CAD build for the part. Positions are in the model's coordinates, mm. Give positions to 0.01 mm unless a question says otherwise; leave off trailing zeros. Write each loop counter-clockwise with the first axis right and the second up, starting at its lowest first coordinate (ties: lowest second). Pieces come first, ordered by that corner, then holes. Notation, with made-up numbers: (-6.5, -22.75) - (40.5, -22.75) arc R25 cw to (40.5, 12.25) - close; hole circle Ø5 at (5, 49). An arc over 180 degrees is marked (long way). Answer as a JSON object with one key per item and string values.
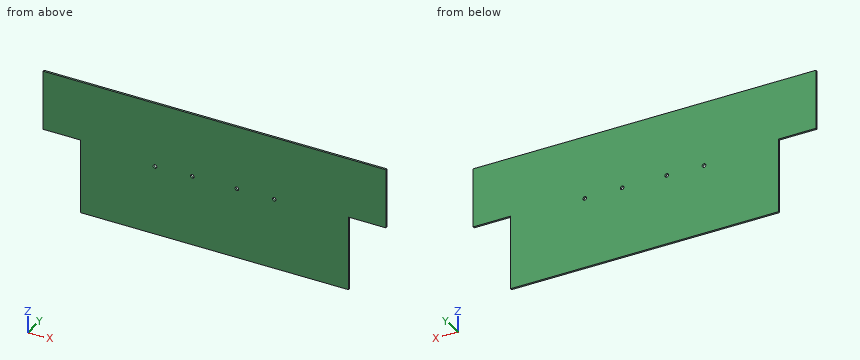
from build123d import *

# Parameters (mm, degrees)
BOSS_EXTRUDE1_DEPTH         = 3.175
F_1_4_0_25_DIAMETER_HOLE1_D = 6.35


with BuildPart() as part:
    # Sketch1 → Boss-Extrude1 (new body)
    with BuildSketch(Plane.XZ.offset(25.4)):
        Polygon((292.1, -215.9), (292.1, -114.3), (0, -114.3), (0, -342.9), (228.6, -342.9), (228.6, -215.9), align=None)
        Polygon((0, -342.9), (0, -114.3), (-292.1, -114.3), (-292.1, -215.9), (-228.6, -215.9), (-228.6, -342.9), align=None)
    extrude(amount=BOSS_EXTRUDE1_DEPTH)

    # 1/4 (0.25) Diameter Hole1 (through all)
    with Locations(Plane(origin=(0, -25.4, 0), x_dir=(1, 0, 0), z_dir=(0, 1, 0))):
        with Locations((-37.935064693, 223.17071982), (-101.416445229, 224.708356097), (38.1, 222.25), (101.6, 222.25)):
            Hole(F_1_4_0_25_DIAMETER_HOLE1_D / 2)


solid = part.part
(1) Flat gauge pins, fed straight in: P1, Ø1, axis at y = -27, z = -254.5, coming from the -X side; P2, Ø5, axis at x = 101.6, z = -222.25, coming from the +Y side. Where does each tip first touch, or does it go through?
Answer key:
{"P1": "stops at x = -228.6", "P2": "passes through"}
(2) Probe L1, parallel to X at y = -27.2, z = -222.25 (1 decimal); L2, parallel to Z at x = 38.1, y = -26.75 (3 decimals); L3, parallel to X at y = -26.85, z = -315.5. List the from-to ranges inside material, lowest first. Write a range as [from, to].
Answer key:
{"L1": "x = [-228.6, -103.4], [-99.4, -41], [-34.9, 34.9], [41.3, 98.4], [104.8, 228.6]", "L2": "z = [-342.9, -225.425], [-219.075, -114.3]", "L3": "x = [-228.6, 228.6]"}
(3) Saw through at B-B, the plane z = -291.5. Give the cut face in (x, y) (3 decimals).
Answer key:
{"outline": "(-228.6, -28.575) - (228.6, -28.575) - (228.6, -25.4) - (-228.6, -25.4) - close"}
(4) Saw through at A-A, the plane y = -26.8. Give the cut face in (x, z) (3 decimals), and give its area (3 significant figures).
Answer key:
{"outline": "(-292.1, -215.9) - (-228.6, -215.9) - (-228.6, -342.9) - (228.6, -342.9) - (228.6, -215.9) - (292.1, -215.9) - (292.1, -114.3) - (-292.1, -114.3) - close; hole circle Ø6.35 at (-101.416, -224.708); hole circle Ø6.35 at (-37.935, -223.171); hole circle Ø6.35 at (38.1, -222.25); hole circle Ø6.35 at (101.6, -222.25)", "area": "117,000 mm²"}
